from build123d import *

# Parameters (mm, degrees)
SKETCH1_W                    = 20
SKETCH1_H                    = 20
BASE_FLANGE1_DEPTH           = 1.5
EDGE_FLANGE1_STRIP_W         = 7.4732
EDGE_FLANGE1_STRIP_H         = 1.5
EDGE_FLANGE1_STRIP_CUT_DEPTH = 20
EDGE_FLANGE1_DEPTH           = 20
EDGE_FLANGE2_START           = -16.736526946
EDGE_FLANGE2_DEPTH           = 20
EDGE_FLANGE2_2_DEPTH         = 20
CUT_EXTRUDE1_DEPTH           = 30.323545381
CUT_EXTRUDE2_DEPTH           = 10


# Read off the part's stored shape, not the designer's step: Edge-Flange2
# Sheet-metal steps are written as plain solids
with BuildPart() as part:
    # Sketch1 → Base-Flange1 (new body)
    with BuildSketch(Plane.XY):
        with Locations((4.191616766, -6.736526946)):
            Rectangle(SKETCH1_W, SKETCH1_H)
    extrude(amount=-BASE_FLANGE1_DEPTH)

    # Edge-Flange1 strip (across the edge) → Edge-Flange1 strip cut (cut)
    with BuildSketch(Plane(origin=(-5.808383234, 3.263473054, 0), x_dir=(1, 0, 0), z_dir=(0, -1, 0))):
        with Locations((-1.5, -0.75)):
            Rectangle(EDGE_FLANGE1_STRIP_W, EDGE_FLANGE1_STRIP_H)
    extrude(amount=EDGE_FLANGE1_STRIP_CUT_DEPTH, mode=Mode.SUBTRACT)

    # Edge-Flange1 section (across the edge) → Edge-Flange1 (add)
    with BuildSketch(Plane(origin=(-5.808383234, 3.263473054, 0), x_dir=(1, 0, 0), z_dir=(0, -1, 0))):
        with BuildLine():
            Line((0, 0.7366), (0, 8.03))
            Line((0, 8.03), (1.5, 8.03))
            Line((1.5, 8.03), (1.5, 0.7366))
            ThreePointArc((1.5, 0.7366), (1.715745145, 0.215745145), (2.2366, 0))
            Line((2.2366, 0), (2.2366, -1.5))
            ThreePointArc((2.2366, -1.5), (0.655084973, -0.844915027), (0, 0.7366))
        make_face()
    extrude(amount=EDGE_FLANGE1_DEPTH)

    # Edge-Flange2 outline → Edge-Flange2 (cut)
    with BuildSketch(Plane(origin=(0, 0, 0), x_dir=(1, 0, 0), z_dir=(0, 1, 0)).offset(EDGE_FLANGE2_START)):
        with BuildLine():
            ThreePointArc((-4.308383234, -5.603569946), (-4.478634271, -6.459479711), (-4.963468207, -7.185084973))
            Line((-4.963468207, -7.185084973), (-5.808383234, -8.03))
            Line((-5.808383234, -8.03), (-4.308383234, -8.03))
            Line((-4.308383234, -8.03), (-4.308383234, -5.603569946))
        make_face()
    extrude(amount=EDGE_FLANGE2_DEPTH, mode=Mode.SUBTRACT)

    # Edge-Flange2 2 outline → Edge-Flange2 2 (add)
    with BuildSketch(Plane(origin=(0, 0, 0), x_dir=(1, 0, 0), z_dir=(0, 1, 0)).offset(EDGE_FLANGE2_START)):
        with BuildLine():
            Line((-14.582644764, -16.804261531), (-5.808383234, -8.03))
            Line((-5.808383234, -8.03), (-5.808383234, -5.603569946))
            ThreePointArc((-5.808383234, -5.603569946), (-5.86445357, -5.885454563), (-6.024128379, -6.124424801))
            Line((-6.024128379, -6.124424801), (-15.643304936, -15.743601359))
            Line((-15.643304936, -15.743601359), (-14.582644764, -16.804261531))
        make_face()
    extrude(amount=EDGE_FLANGE2_2_DEPTH)

    # Sketch12 → Cut-Extrude1 (cut, through all)
    with BuildSketch(Plane(origin=(0, 0, -1.5), x_dir=(-1, 0, 0), z_dir=(0, 0, -1))):
        with BuildLine():
            Line((-2.925555282, -14.486526946), (-10.71929847, -14.486526946))
            ThreePointArc((-10.71929847, -14.486526946), (-12.46929847, -12.736526946), (-10.71929847, -10.986526946))
            Line((-10.71929847, -10.986526946), (-2.925555282, -10.986526946))
            ThreePointArc((-2.925555282, -10.986526946), (-1.175555282, -12.736526946), (-2.925555282, -14.486526946))
        make_face()
        with BuildLine():
            Line((-2.925555282, -2.486526946), (-10.71929847, -2.486526946))
            ThreePointArc((-10.71929847, -2.486526946), (-12.46929847, -0.736526946), (-10.71929847, 1.013473054))
            Line((-10.71929847, 1.013473054), (-2.925555282, 1.013473054))
            ThreePointArc((-2.925555282, 1.013473054), (-1.175555282, -0.736526946), (-2.925555282, -2.486526946))
        make_face()
    extrude(amount=-CUT_EXTRUDE1_DEPTH, mode=Mode.SUBTRACT)

    # Sketch13 → Cut-Extrude2 (cut)
    with BuildSketch(Plane(origin=(0.050148211, 0, 0.050148211), x_dir=(-0.7071067811865465, 0, 0.7071067811865487), z_dir=(-0.7071067811865487, 0, -0.7071067811865465))):
        with BuildLine():
            Line((17.152424018, -13.736526946), (17.152424018, 0.263473054))
            ThreePointArc((17.152424018, 0.263473054), (18.902424018, 2.013473054), (20.652424018, 0.263473054))
            Line((20.652424018, 0.263473054), (20.652424018, -13.736526946))
            ThreePointArc((20.652424018, -13.736526946), (18.902424018, -15.486526946), (17.152424018, -13.736526946))
        make_face()
    extrude(amount=-CUT_EXTRUDE2_DEPTH, mode=Mode.SUBTRACT)


solid = part.part
Design review of the part built by this model. Coordinates are the model's own, in mm. A direction names the side the tool comes from. Coordinates: 2 decimals unless noted, no trailing zeros. Write each loop counter-clockwise with the first axis right and the second up, starting at its lowest first coordinate (ties: lowest second). Pieces come first, ordered by that corner, then holes. Notation, with made-up numbers: (7, -15.5) - (21, -15.5) arc R7 cw to (21, -2.5) - close; hole circle Ø9 at (73, 80.5). An arc over 180 degrees is marked (long way). One line per item, written item: value.
1) Mouldability with a two-part tool opening along X and no side actions: class faces 1 (the face through (-15.12, -6.877, 16.267)), 2 (the face through (7, -14.487, -1)), 3 (the face through (5, -7, 0)) as +X half, -X half, draft (parallel to the pull), parting line (faces both ways), or undercut.
Answer sheet:
face 1: -X half
face 2: undercut
face 3: draft
2) Add section A-A (y = -6). State the section outline as (x, z) points, plus the area to 3 significant figures.
Answer sheet:
outline: (-15.64, 15.74) - (-14.55, 14.65) - (-13.49, 15.71) - (-14.58, 16.8) - close; (-12.08, 12.18) - (-6.02, 6.12) arc R0.74 cw to (-5.81, 5.6) - (-5.81, 0.74) arc R2.24 ccw to (-3.57, -1.5) - (14.19, -1.5) - (14.19, 0) - (-3.57, 0) arc R0.74 cw to (-4.31, 0.74) - (-4.31, 5.6) arc R2.24 ccw to (-4.96, 7.19) - (-11.02, 13.24) - close
area: 54.4 mm2
3) Add section D-D (z = 4.5). State the section outline as (x, y) points.
Answer sheet:
outline: (-5.81, -16.74) - (-4.31, -16.74) - (-4.31, 3.26) - (-5.81, 3.26) - close
4) Insertion check: pin 1 (5.5 mm diameter, centred on x = 5.5, y = -6.5, fed in from +Z); pin 2 (1 mm diameter, centred on y = -1, z = 4.5, fed in from -X); pin 3 (10 mm diameter, centred on y = -13, z = 12, fed in from -X). Each pin has a flat end and moves straight along its axis. Give the tip position at first contact, or say it passes through.
Answer sheet:
pin 1: stops at z = 0
pin 2: stops at x = -5.81
pin 3: stops at x = -15.64
5) To check wall thickness, follow probe 1 along X at (y, z) = (-2.25, 2); probe 2 along Z at (x, y) = (3, -3.5); probe 3 along X at (y, z) = (-8.75, 11). State the ranges of each line that lie inside material, in increasing order.
Answer sheet:
probe 1: x = -5.81 to -4.31
probe 2: z = -1.5 to 0
probe 3: x = -10.9 to -8.78
6) For faces 4 (the face through (-12.766, 2.013, 13.912)), 5 (the face through (-14.03, -6.639, 15.177)), 6 (the face through (-5.808, -7, 3)), 7 (the face through (1.176, -12.698, -0.76)), list the 3-axis set-ups (+Z, -Z, +X, -X, +Y, -Y) from which the entire face can be reached by the end or side of a thin tool; tool diameter is ignored.
Answer sheet:
face 4: none
face 5: -Z, +X
face 6: -Z, -X, +Y, -Y
face 7: +Z, -Z
7) Add section C-C (y = -13). State the section outline as (x, z) points.
Answer sheet:
outline: (-15.64, 15.74) - (-14.55, 14.65) - (-13.49, 15.71) - (-14.58, 16.8) - close; (-12.08, 12.18) - (-6.02, 6.12) arc R0.74 cw to (-5.81, 5.6) - (-5.81, 0.74) arc R2.24 ccw to (-3.57, -1.5) - (1.2, -1.5) - (1.2, 0) - (-3.57, 0) arc R0.74 cw to (-4.31, 0.74) - (-4.31, 5.6) arc R2.24 ccw to (-4.96, 7.19) - (-11.02, 13.24) - close; (12.45, -1.5) - (14.19, -1.5) - (14.19, 0) - (12.45, 0) - close
8) Add section B-B (x = 9.25). State the section outline as (y, z) points, plus the area to 3 significant figures.
Answer sheet:
outline: (-16.74, -1.5) - (-14.49, -1.5) - (-14.49, 0) - (-16.74, 0) - close; (-10.99, -1.5) - (-2.49, -1.5) - (-2.49, 0) - (-10.99, 0) - close; (1.01, -1.5) - (3.26, -1.5) - (3.26, 0) - (1.01, 0) - close
area: 19.5 mm2
